```python
from build123d import *

# Parameters (mm, degrees)
F1_DEPTH = 30
F3_D     = 8
F5_D     = 4


with BuildPart() as f1:
    # F0 (on Front) → F1 (new body)
    with BuildSketch(Plane.XZ):
        Polygon((17, 0), (-17, 0), (-17, -18), (-8, -18), (-4, -22), (4, -22), (8, -18), (17, -18), align=None)
    extrude(amount=F1_DEPTH)

    # F3 (through all)
    with Locations(Plane(origin=(0, 0, 0), x_dir=(-1, 0, 0), z_dir=(0, 1, 0))):
        with Locations((0, -11)):
            Hole(F3_D / 2)

    # F5 (through all)
    with Locations(Plane.XY):
        with Locations((12, -24), (12, -6), (-12, -6), (-12, -24)):
            Hole(F5_D / 2)


solid = f1.part
```
Here's how the part is built. I have some questions about the finished solid (model axes, mm). A direction names the side the tool comes from. Give positions to 0.01 mm unless a question says otherwise; leave off trailing zeros. Order: outer loops, then holes, each group sorted by start corner. A loop starts at its lowest first (then second) coordinate and runs counter-clockwise, first axis right, second up. Notation, with made-up numbers: (-15, -7) - (1, -7) arc R21 ccw to (1, 24) - close; hole circle Ø5 at (66, -7.5). An arc over 180 degrees is marked (long way). Answer as a JSON object with one key per item and string values. Group by question number.
Item 1: If we section it at B-B on y = -6: Please give me the cut outline in (x, z), and give its area (3 significant figures).
Item 2: If we section it at D-D on x = -12: Please give me the cut outline in (y, z).
Item 3: If we section it at A-A on x = 0: Please give me the cut outline in (y, z).
Item 4: If we section it at C-C on z = -11: Please give me the cut outline in (x, y), and give its area (3 significant figures).
Item 5: For P1, Ø5, axis at x = 12, y = -6, coming from the -Z side; P2, Ø3.5, axis at x = -12, y = -24, coming from the +Z side, each with a flat end and sliding along its axis, tell me the tip position at first contact or that it passes through.
Item 6: Which directions (+Z, -Z, +X, -X, +Y, -Y) give clear straight access to the entire face, cutting with the end or side of a thin tool? Please do faces 4 (the flat face through (-13, -15, -18)), 5 (the cylindrical face through (-0.867, -15.21, -14.905)).
Item 7: If we mould it in two halves opening along Y, with no side actions, what happens to faces 1 (the flat face through (12, -15, -18)), 2 (the cylindrical face through (-10, -24, -9)), 3 (the flat face through (0, 0, -6))? For each: pulls with the +Y half, pulls with the -Y half, needs draft (parallel to the pull), parting line crosses it, or undercut.
Item 8: Please list where these lines run through material, in increasing order: probe 1 along Y at (x, z) = (-12, -12.5); probe 2 along Z at (x, y) = (0, -15.5); probe 3 along Z at (x, y) = (-14.5, -11.5).
Result set:
{
 "1": {"outline": "(-17, -18) - (-14, -18) - (-14, 0) - (-17, 0) - close; (-10, -18) - (-8, -18) - (-4, -22) - (4, -22) - (8, -18) - (10, -18) - (10, 0) - (-10, 0) - close; (14, -18) - (17, -18) - (17, 0) - (14, 0) - close; hole circle Ø8 at (0, -11)", "area": "466 mm²"},
 "2": {"outline": "(-30, -18) - (-26, -18) - (-26, 0) - (-30, 0) - close; (-22, -18) - (-8, -18) - (-8, 0) - (-22, 0) - close; (-4, -18) - (0, -18) - (0, 0) - (-4, 0) - close"},
 "3": {"outline": "(-30, -22) - (0, -22) - (0, -15) - (-30, -15) - close; (-30, -7) - (0, -7) - (0, 0) - (-30, 0) - close"},
 "4": {"outline": "(-17, -30) - (-4, -30) - (-4, 0) - (-17, 0) - close; (4, -30) - (17, -30) - (17, 0) - (4, 0) - close; hole circle Ø4 at (-12, -24); hole circle Ø4 at (-12, -6); hole circle Ø4 at (12, -24); hole circle Ø4 at (12, -6)", "area": "730 mm²"},
 "5": {"P1": "z = -18", "P2": "through"},
 "6": {"face 4": "-Z, -X, +Y, -Y", "face 5": "+Y, -Y"},
 "7": {"face 1": "needs draft", "face 2": "undercut", "face 3": "pulls with the +Y half"},
 "8": {"probe 1": "-30 to -26, -22 to -8, -4 to 0", "probe 2": "-22 to -15, -7 to 0", "probe 3": "-18 to 0"}
}
